Build history of the part. All positions in model axes, mm. Face numbers are marked on the shaded views. Round coordinates to 2 decimals unless told otherwise and drop trailing zeros. Loops run counter-clockwise (first coordinate to the right, second up) from the corner with the lowest first, then second, coordinate; pieces in that order, holes last. Notation, with made-up numbers: (11.25, 20) - (57.25, 20) arc R17 ccw to (57.25, 48) - close; hole circle Ø2 at (10.25, 83.5). An arc over 180 degrees is marked (long way). Put each result on its own line as item: value. Start each with the question number.
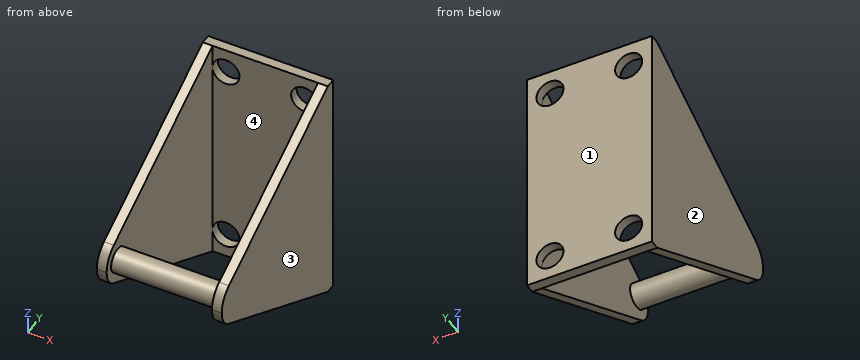
from build123d import *

# Parameters (mm, degrees)
BOSS_EXTRUDE1_DEPTH          = 47.752
CUT_EXTRUDE1_DEPTH           = 47.752
CUT_EXTRUDE1_DEPTH_BACK      = 47.752
BOSS_EXTRUDE6_START          = -10.7
SKETCH3_R                    = 2.5
BOSS_EXTRUDE6_DEPTH          = 10.7
SKETCH3_2_R                  = 2.5
BOSS_EXTRUDE7_DEPTH          = 10.7
M5_START                     = -2
M5_CLEARANCE_HOLE1_OUTLINE_R = 2.75
M5_CLEARANCE_HOLE1_DEPTH     = 2


# Read off the part's stored shape, not the designer's step: M5 Clearance Hole1
with BuildPart() as part:
    # Sketch1 → Boss-Extrude1 (new body)
    with BuildSketch(Plane.XY):
        Polygon((-12.7, -41.275), (-12.7, 0), (12.7, 0), (12.7, -41.275), (10.7, -41.275), (10.7, -2), (-10.7, -2), (-10.7, -41.275), align=None)
    extrude(amount=BOSS_EXTRUDE1_DEPTH)

    # Sketch2 → Cut-Extrude1 (cut, two sides: drawn at the far end of the back side and taken through both)
    with BuildSketch(Plane(origin=(0, 0, 0), x_dir=(0, 0, -1), z_dir=(1, 0, 0)).offset(-CUT_EXTRUDE1_DEPTH_BACK)):
        with BuildLine():
            Line((-23.876, -42.10871549), (-23.876, -41.275))
            ThreePointArc((-23.876, -41.275), (-26.451700932, -40.560529688), (-28.291297125, -38.621305883))
            Line((-28.291297125, -38.621305883), (-47.752, -2))
            Line((-47.752, -2), (-47.752, -42.10871549))
            Line((-47.752, -42.10871549), (-23.876, -42.10871549))
        make_face()
        with BuildLine():
            Line((0, -42.10871549), (0, -2))
            Line((0, -2), (-19.460702875, -38.621305883))
            ThreePointArc((-19.460702875, -38.621305883), (-21.300299068, -40.560529688), (-23.876, -41.275))
            Line((-23.876, -41.275), (-23.876, -42.10871549))
            Line((-23.876, -42.10871549), (0, -42.10871549))
        make_face()
    extrude(amount=CUT_EXTRUDE1_DEPTH + CUT_EXTRUDE1_DEPTH_BACK, mode=Mode.SUBTRACT)

    # Sketch3 → Boss-Extrude6 (add)
    with BuildSketch(Plane(origin=(0, 0, 0), x_dir=(0, 0, -1), z_dir=(1, 0, 0)).offset(BOSS_EXTRUDE6_START)):
        with Locations((-23.876, -37.128004449)):
            Circle(SKETCH3_R)
    extrude(amount=BOSS_EXTRUDE6_DEPTH)

    # Sketch3<2> → Boss-Extrude7 (add)
    with BuildSketch(Plane(origin=(0, 0, 0), x_dir=(0, 0, -1), z_dir=(1, 0, 0))):
        with Locations((-23.876, -37.128004449)):
            Circle(SKETCH3_2_R)
    extrude(amount=BOSS_EXTRUDE7_DEPTH)

    # M5 Clearance Hole1 outline → M5 Clearance Hole1 (cut)
    with BuildSketch(Plane(origin=(0, 0, 0), x_dir=(1, 0, 0), z_dir=(0, 1, 0)).offset(M5_START)):
        with Locations((8, -5)):
            Circle(M5_CLEARANCE_HOLE1_OUTLINE_R)
        with Locations((8, -42.752)):
            Circle(M5_CLEARANCE_HOLE1_OUTLINE_R)
        with Locations((-8, -42.752)):
            Circle(M5_CLEARANCE_HOLE1_OUTLINE_R)
        with Locations((-8, -5)):
            Circle(M5_CLEARANCE_HOLE1_OUTLINE_R)
    extrude(amount=M5_CLEARANCE_HOLE1_DEPTH, mode=Mode.SUBTRACT)


solid = part.part
1) Slice it at B-B, the plane x = 8. Write the cut outline in (y, z), and give its area (3 significant figures).
2) Slice it at A-A, the plane y = -23.5. Write the cut outline in (x, z).
3) Slice it at C-C, the plane z = 15. Write the cut outline in (x, y).
4) Drill centre lines: line 1 (Z direction, x = -8, y = -1.45); line 2 (X direction, y = -0.8, z = 5); line 3 (X direction, y = -15.5, z = 11.5). Where is each one in solid material? Low to high. Write a range as [from, to].
5) Slice it at D-D, the plane y = -35.5. Write the cut outline in (x, z).
6) Pull direction X, two halves, no side cores. Call the marked faces 1, 2, 3 and 4: pulls with the +X half, pulls with the -X half, needs draft (parallel to the pull), parting line crosses it, or undercut.
7) Drop flat-ended pins along their axis: pin 1 Ø10 at (x, y) = (1, -26) entering from -Z; pin 2 Ø2 at (x, z) = (3, 14) entering from +Y; pin 3 Ø10.5 at (x, z) = (-1.5, 35.5) entering from -Y; pin 4 Ø12 at (x, y) = (-8.5, -18) entering from -Z. Give the stop position or say it passes through.
Taken from the geometry:
1. outline: circle Ø5 at (-37.13, 23.88); (-2, 0) - (0, 0) - (0, 2.25) - (-2, 2.25) - close; (-2, 7.75) - (0, 7.75) - (0, 40) - (-2, 40) - close; (-2, 45.5) - (0, 45.5) - (0, 47.75) - (-2, 47.75) - close
1. area: 93.1 mm2
2. outline: (-12.7, 11.43) - (-10.7, 11.43) - (-10.7, 36.33) - (-12.7, 36.33) - close; (10.7, 11.43) - (12.7, 11.43) - (12.7, 36.33) - (10.7, 36.33) - close
3. outline: (-12.7, -30.23) - (-10.7, -30.23) - (-10.7, -2) - (10.7, -2) - (10.7, -30.23) - (12.7, -30.23) - (12.7, 0) - (-12.7, 0) - close
4. line 1: z = [0, 2.25], [7.75, 40], [45.5, 47.75]
4. line 2: x = [-12.7, -10.75], [-5.25, 5.25], [10.75, 12.7]
4. line 3: x = [-12.7, -10.7], [10.7, 12.7]
5. outline: (-12.7, 17.8) - (-10.7, 17.8) - (-10.7, 21.98) - (10.7, 21.98) - (10.7, 17.8) - (12.7, 17.8) - (12.7, 29.95) - (10.7, 29.95) - (10.7, 25.77) - (-10.7, 25.77) - (-10.7, 29.95) - (-12.7, 29.95) - close
6. face 1: needs draft
6. face 2: pulls with the -X half
6. face 3: pulls with the +X half
6. face 4: undercut
7. pin 1: passes through
7. pin 2: stops at y = 0
7. pin 3: stops at y = -2
7. pin 4: stops at z = 5.54
